```python
from build123d import *

# Parameters (mm, degrees)
F0_R      = 2
F0_R_2    = 0.1
F1_DEPTH  = 12
F0_R_3    = 1.5
F2_DEPTH  = 15
F4_R      = 0.1
F5_DEPTH  = 2
F6_COUNT  = 3
F5_FACE_R = 0.1
F6_FACE_R = 0.1
F7_DEPTH  = 4.2


# Not quite as in the source:
# - a fillet or chamfer that OpenCascade refuses, or shapes differently, is made with other operations: its cross-section is extruded or revolved along the edge and cut away or added


with BuildPart() as f1:
    # F0 (on Front) → F1 (new body)
    with BuildSketch(Plane.XZ):
        with BuildLine():
            ThreePointArc((4.7997142496, 7.1366126269), (-12.410762485, -13.4329699503), (13.278817402, -5.728833265))
            ThreePointArc((13.278817402, -5.728833265), (12.9087772386, -2.5313037732), (11.8182181375, 0.4971950993))
            Line((11.8182181375, 0.4971950993), (-2.2800283653, 0.4971950993))
            Line((-2.2800283653, 0.4971950993), (-3.8388741325, 3.1971951693))
            Line((-3.8388741325, 3.1971951693), (-2.2800283653, 5.8971952394))
            Line((-2.2800283653, 5.8971952394), (0.8376631692, 5.8971952394))
            Line((0.8376631692, 5.8971952394), (2.174251278, 3.5821567261))
            ThreePointArc((2.174251278, 3.5821567261), (3.4311500139, 5.4006249736), (4.7997142496, 7.1366126269))
        make_face()
        with Locations((-0.721182598, -5.728833265)):
            Circle(F0_R, mode=Mode.SUBTRACT)
        with BuildLine():
            Line((-2.2800283653, 0.4971950993), (11.8182181375, 0.4971950993))
            ThreePointArc((11.8182181375, 0.4971950993), (8.8998388381, 4.4415131659), (4.7997142496, 7.1366126269))
            ThreePointArc((4.7997142496, 7.1366126269), (3.4311500139, 5.4006249736), (2.174251278, 3.5821567261))
            Line((2.174251278, 3.5821567261), (0.8376631692, 5.8971952394))
            Line((0.8376631692, 5.8971952394), (-2.2800283653, 5.8971952394))
            Line((-2.2800283653, 5.8971952394), (-3.8388741325, 3.1971951693))
            Line((-3.8388741325, 3.1971951693), (-2.2800283653, 0.4971950993))
        make_face()
        with Locations((-0.7538866513, 3.197135257)):
            Circle(F0_R_2, mode=Mode.SUBTRACT)
    extrude(amount=F1_DEPTH)

    # F0 (on Front) → F2 (join)
    with BuildSketch(Plane.XZ):
        with Locations((-0.721182598, -5.728833265)):
            Circle(F0_R)
        with Locations((-0.721182598, -5.728833265)):
            Circle(F0_R_3, mode=Mode.SUBTRACT)
    extrude(amount=F2_DEPTH)

    # F3: chamfer of 9 x 11.5194746897 on 1 edges, made by hand

    # F3_s1 → F3_t2 (revolve, cut)
    with BuildSketch(Plane.XY.offset(-5.728833265)):
        Polygon((12.2982920917, 0), (0.778817402, -9), (0.778817402, 0), align=None)
    revolve(axis=Axis((-0.721182598, 0, -5.728833265), (0, -1, 0)), mode=Mode.SUBTRACT)

    # F6: F5 ×3 about axis
    f6_axis = Axis((-0.721182598, 0, -5.728833265), (0, -1, 0))


with BuildPart() as f5:
    # F4 (on face) → F5 (new body)
    with BuildSketch(Plane.XZ.offset(12)):
        with BuildLine():
            Line((-2.2800283653, 0.4971950993), (11.8182181375, 0.4971950993))
            ThreePointArc((11.8182181375, 0.4971950993), (8.8998388381, 4.4415131659), (4.7997142496, 7.1366126269))
            ThreePointArc((4.7997142496, 7.1366126269), (3.4311500139, 5.4006249736), (2.174251278, 3.5821567261))
            Line((2.174251278, 3.5821567261), (0.8376631692, 5.8971952394))
            Line((0.8376631692, 5.8971952394), (-2.2800283653, 5.8971952394))
            Line((-2.2800283653, 5.8971952394), (-3.8388741325, 3.1971951693))
            Line((-3.8388741325, 3.1971951693), (-2.2800283653, 0.4971950993))
        make_face()
        with Locations((-0.7538866513, 3.197135257)):
            Circle(F4_R, mode=Mode.SUBTRACT)
    extrude(amount=F5_DEPTH)


with BuildPart() as f1_1:
    add(f1.part)
    for i in range(1, F6_COUNT):
        add(f5.part.rotate(f6_axis, i * 360 / F6_COUNT))


with BuildPart() as f7_tool:
    # F5_face (on face) + F6_face (on face) → F7 (new body)
    with BuildSketch(Plane(origin=(3.5829132763, -14, 3.0354703716), x_dir=(1, 0, 0), z_dir=(0, -1, 0))):
        with BuildLine():
            Line((-5.8629416416, 2.8617248677), (-7.4217874088, 0.1617247977))
            Line((-7.4217874088, 0.1617247977), (-5.8629416416, -2.5382752723))
            Line((-5.8629416416, -2.5382752723), (8.2353048612, -2.5382752723))
            ThreePointArc((8.2353048612, -2.5382752723), (5.3169255618, 1.4060427943), (1.2168009733, 4.1011422553))
            ThreePointArc((1.2168009733, 4.1011422553), (-0.1517632624, 2.365154602), (-1.4086619983, 0.5466863545))
            Line((-1.4086619983, 0.5466863545), (-2.7452501071, 2.8617248677))
            Line((-2.7452501071, 2.8617248677), (-5.8629416416, 2.8617248677))
        make_face()
        with Locations((-4.3367999276, 0.1616648853)):
            Circle(F5_FACE_R, mode=Mode.SUBTRACT)
    with BuildSketch(Plane(origin=(4.7168790606, -14, -13.8384414508), x_dir=(1, 0, 0), z_dir=(0, -1, 0))):
        with BuildLine():
            Line((5.4097972549, 3.6465939687), (3.8509514876, 6.3465940387))
            Line((3.8509514876, 6.3465940387), (0.7332599531, 6.3465940387))
            Line((0.7332599531, 6.3465940387), (-6.3158632983, -5.8628455816))
            ThreePointArc((-6.3158632983, -5.8628455816), (-1.4407940022, -5.3076140037), (2.943292891, -3.1043516819))
            ThreePointArc((2.943292891, -3.1043516819), (2.1241656004, -1.0511464604), (1.17777527, 0.9465938986))
            Line((1.17777527, 0.9465938986), (3.8509514876, 0.9465938986))
            Line((3.8509514876, 0.9465938986), (5.4097972549, 3.6465939687))
        make_face()
        with Locations((2.3084058614, 3.6749464658)):
            Circle(F6_FACE_R, mode=Mode.SUBTRACT)
        with BuildLine():
            Line((-14.7270748049, 0.9465938986), (-11.6093832704, 0.9465938986))
            Line((-11.6093832704, 0.9465938986), (-10.0505375032, 3.6465939687))
            Line((-10.0505375032, 3.6465939687), (-17.0996607546, 15.8560335889))
            ThreePointArc((-17.0996607546, 15.8560335889), (-19.0563507512, 11.3564839444), (-19.3403130559, 6.4581221616))
            ThreePointArc((-19.3403130559, 6.4581221616), (-17.1526215296, 6.1409045934), (-14.9493324633, 5.9616324819))
            Line((-14.9493324633, 5.9616324819), (-16.2859205721, 3.6465939687))
            Line((-16.2859205721, 3.6465939687), (-14.7270748049, 0.9465938986))
        make_face()
        with Locations((-13.1518251254, 3.6183013839)):
            Circle(F6_FACE_R, mode=Mode.SUBTRACT)
    extrude(amount=-F7_DEPTH)


with BuildPart() as f1_2:
    add(f1_1.part)

    # F7: cut by f7_tool
    add(f7_tool.part, mode=Mode.SUBTRACT)


with BuildPart() as f5_1:
    add(f5.part)

    # F7: cut by f7_tool
    add(f7_tool.part, mode=Mode.SUBTRACT)


solid = f1_2.part
```
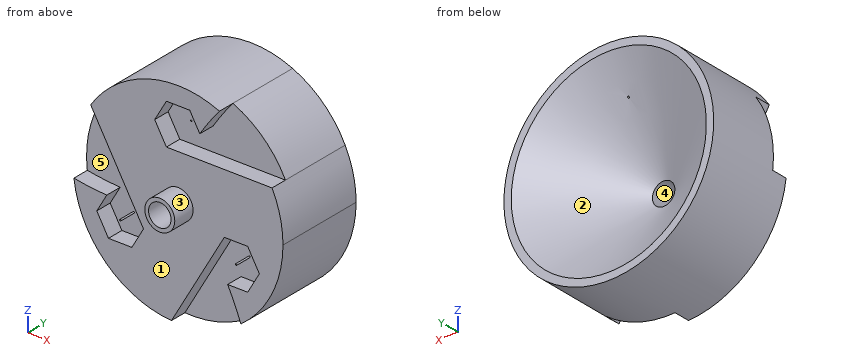
Geometry: final body of the model. Coordinates: model frame, mm. Face numbers are marked on the shaded views. A direction names the side the tool comes from. Coordinates: 2 decimals unless noted, no trailing zeros. Loops run counter-clockwise (first coordinate to the right, second up) from the corner with the lowest first, then second, coordinate; pieces in that order, holes last. Notation, with made-up numbers: M 4.25,81 L 33.25,81 A3 cw 33.25,85 Z; hole C 2.25,4 d3. An arc over 180 degrees is marked long. Put each result on its own line as item: value.
(1) Cut plane D-D on y = -5.75. Return the cut outline in (x, z), then the cut area to 3 significant figures.
Answer sheet:
outline: C -0.72,-5.73 d28; hole C -0.72,-5.73 d11.32; hole C -0.75,3.2 d0.2
area: 515 mm^2
(2) Cut plane C-C on y = -13.25. Return the cut outline in (x, z), then the cut area to 3 significant figures.
Answer sheet:
outline: C -0.72,-5.73 d4; hole C -0.72,-5.73 d3
area: 5.50 mm^2
(3) Access query for the marked faces 4 and 5. Directions: +Z, -Z, +X, -X, +Y, -Y. A direction counts if a zero-diameter tool reaches every point of the face in a straight line with its end or side. Return the directions, or none.
Answer sheet:
face 4: +Y, -Y
face 5: -Y
(4) Draft query along Z for the marked faces 1, 2 and 3. Return one class per face: pulls with the +Z half, pulls with the -Z half, needs draft (parallel to the pull), parting line crosses it, or undercut.
Answer sheet:
face 1: needs draft
face 2: undercut
face 3: parting line crosses it
(5) First-contact query: pin 1 (10.5 mm diameter, centred on x = -12, z = -3.5, fed in from -Y); pin 2 (2 mm diameter, centred on x = 8, y = -8.5, fed in from +Z); pin 3 (1.1 mm diameter, centred on x = 0, y = -11.5, fed in from -Z); pin 4 (2.5 mm diameter, centred on x = -0.72, z = -5.73, fed in from +Y). Flat tips, straight axial feed; report the tip coordinate or a pass-through.
Answer sheet:
pin 1: stops at y = -12
pin 2: stops at z = 5.95
pin 3: stops at z = -17.88
pin 4: passes through
(6) Cut plane B-B on y = -7.5. Return the cut outline in (x, z), then the cut area to 3 significant figures.
Answer sheet:
outline: C -0.72,-5.73 d28; hole C -0.72,-5.73 d6.84; hole C -0.75,3.2 d0.2
area: 579 mm^2
(7) Material intervals for probe 1 along X at (y, z) = (-10.5, -12); probe 2 along X at (y, z) = (-11.25, -11); probe 3 along X at (y, z) = (-4.75, -8.25), sorted ascending.
Answer sheet:
probe 1: x = -13.24 to -10.53, -6.38 to 2.85, 9.08 to 11.8
probe 2: x = -13.69 to -11.1, -5.8 to 3.42, 9.66 to 12.25
probe 3: x = -14.49 to -7.19, 5.74 to 13.05
(8) Cut plane A-A on y = -11. Return the cut outline in (x, z), then the cut area to 3 significant figures.
Answer sheet:
outline: M -14.62,-7.38 A14 ccw -1.6,-19.7 L 5.45,-7.49 L 8.57,-7.49 L 10.13,-10.19 L 8.57,-12.89 L 5.89,-12.89 A35.2 cw 7.66,-16.94 A14 ccw 11.82,0.5 L -2.28,0.5 L -3.84,3.2 L -2.28,5.9 L 0.84,5.9 L 2.17,3.58 A35.2 cw 4.8,7.14 A14 ccw -12.38,2.02 L -5.33,-10.19 L -6.89,-12.89 L -10.01,-12.89 L -11.57,-10.19 L -10.23,-7.88 A35.2 cw Z; C -8.43,-10.22 d0.2; C 7.03,-10.16 d0.2; hole C -0.72,-5.73 d3
area: 403 mm^2
